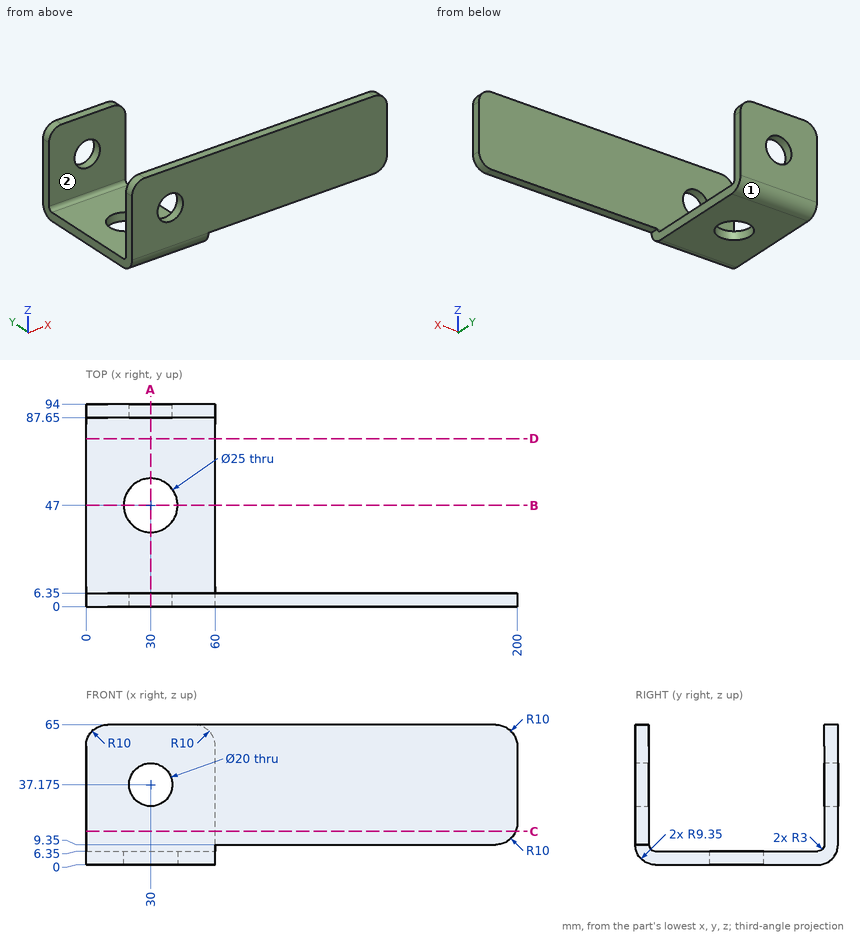
Could you check a few things on this drawing? It's one solid part, dimensions in mm from its lowest x, y, z. A direction names the side the tool comes from. Round coordinates to 2 decimals unless told otherwise and drop trailing zeros. Order: outer loops, then holes, each group sorted by start corner. A loop starts at its lowest first (then second) coordinate and runs counter-clockwise, first axis right, second up. Notation, with made-up numbers: M 0.5,-30 L 39.5,-30 A14 cw 39.5,-16 Z; hole C 61.25,54.5 d11. An arc over 180 degrees is marked long. Return JSON: item names as keys, results as strings. Group by question number.
1. If we section it at D-D on y = 78: List the corners of the cut face in (x, z) for me, then the cut area to 3 significant figures.
2. If we section it at C-C on z = 15.5: List the corners of the cut face in (x, y) for me, then the cut area to 3 significant figures.
3. If we section it at A-A on x = 30: List the corners of the cut face in (y, z) for me (3 decimals).
4. On a 3-axis mill with a long thin cutter (end or side, diameter ignored), from which of +Z, -Z, +X, -X, +Y, -Y can I reach the whole of each face in a straight line? I mean the marked faces 1 and 2. Say none if no direction works.
5. I'm going to push flat-ended pins straight in: pin 1 Ø23 at (x, z) = (30, 37.175) entering from +Y; pin 2 Ø12 at (x, z) = (74, 45) entering from +Y; pin 3 Ø2 at (x, z) = (123.5, 26.5) entering from +Y; pin 4 Ø1.9 at (x, y) = (151.5, 4) entering from -Z. Where does each tip first touch, or does it pass through?
6. If we section it at B-B on y = 47: List the corners of the cut face in (x, z) for me, then the cut area to 3 significant figures.
7. Please list where these lines run through material, in increasing order: probe 1 along Y at (x, z) = (10.5, 41.5); probe 2 along Z at (x, y) = (11, 70.5).
Reply:
{
 "1": {"outline": "M 0,0 L 60,0 L 60,6.35 L 0,6.35 Z", "area": "381 mm^2"},
 "2": {"outline": "M 0,0 L 199.23,0 L 199.23,6.35 L 0,6.35 Z; M 0,87.65 L 60,87.65 L 60,94 L 0,94 Z", "area": "1,650 mm^2"},
 "3": {"outline": "M 0,9.35 A9.35 ccw 9.35,0 L 34.5,0 L 34.5,6.35 L 9.35,6.35 A3 cw 6.35,9.35 L 6.35,27.175 L 0,27.175 Z; M 0,47.175 L 6.35,47.175 L 6.35,65 L 0,65 Z; M 59.5,0 L 84.65,0 A9.35 ccw 94,9.35 L 94,27.175 L 87.65,27.175 L 87.65,9.35 A3 cw 84.65,6.35 L 59.5,6.35 Z; M 87.65,47.175 L 94,47.175 L 94,65 L 87.65,65 Z"},
 "4": {"face 1": "-Z, +X, -X, +Y", "face 2": "+Z, +X, -X"},
 "5": {"pin 1": "y = 94", "pin 2": "y = 6.35", "pin 3": "y = 6.35", "pin 4": "z = 9.35"},
 "6": {"outline": "M 0,0 L 17.5,0 L 17.5,6.35 L 0,6.35 Z; M 42.5,0 L 60,0 L 60,6.35 L 42.5,6.35 Z", "area": "222 mm^2"},
 "7": {"probe 1": "0 to 6.35, 87.65 to 94", "probe 2": "0 to 6.35"}
}
